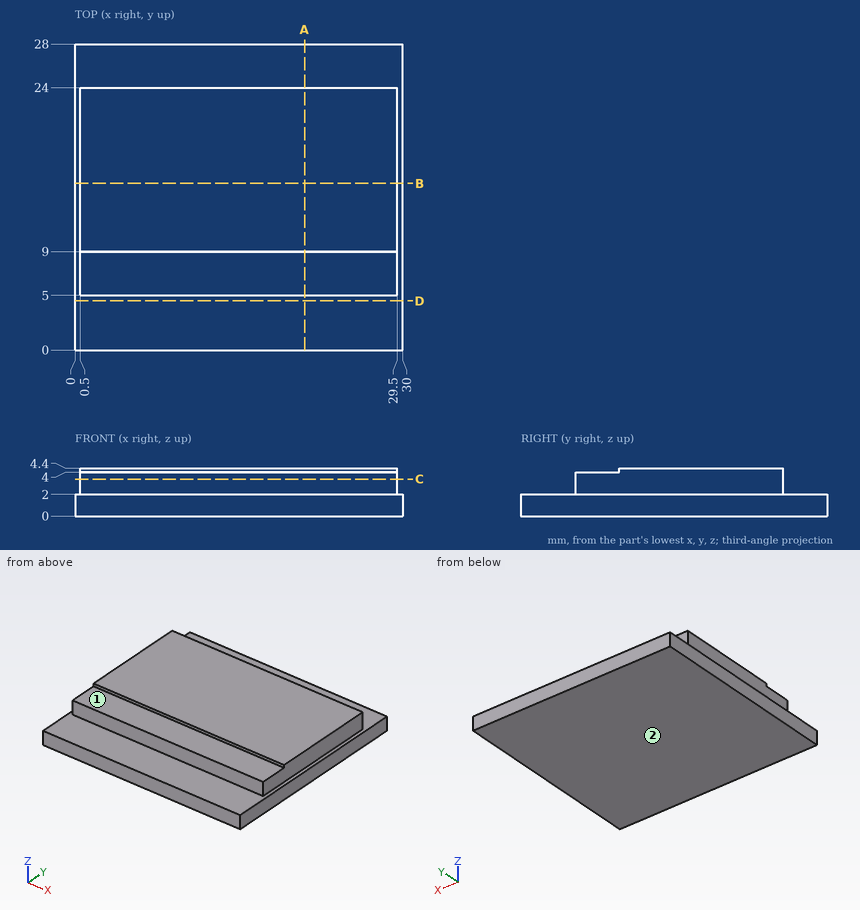
Print and shaded views of the part. All mm, measured from the part's lowest x, y and z. A direction names the side the tool comes from. Give positions to 0.01 mm unless a question says otherwise; leave off trailing zeros. Order: outer loops, then holes, each group sorted by start corner. A loop starts at its lowest first (then second) coordinate and runs counter-clockwise, first axis right, second up. Notation, with made-up numbers: (57, 69.25) - (116, 69.25) arc R6 ccw to (116, 77.25) - close; hole circle Ø2 at (27.5, -1). An arc over 180 degrees is marked (long way). Use a Markdown table: item, result.
1) Saw through at B-B on y = 15.25. List the corners of the cut face in (x, z), plus the area to 3 significant figures.
Checked values:
| item | result |
|---|---|
| outline | (0, 0) - (30, 0) - (30, 2) - (29.5, 2) - (29.5, 4.4) - (0.5, 4.4) - (0.5, 2) - (0, 2) - close |
| area | 130 mm² |
2) Probe L1, parallel to Z at x = 1.5, y = 4.75; L2, parallel to Y at x = 24, z = 3.05; L3, parallel to Y at x = 8.75, z = 4.1. List the from-to ranges inside material, lowest first. Write a range as from..to.
Checked values:
| item | result |
|---|---|
| L1 | 0..2 |
| L2 | 5..24 |
| L3 | 9..24 |
3) Saw through at C-C on z = 3.4. List the corners of the cut face in (x, y).
Checked values:
| item | result |
|---|---|
| outline | (0.5, 5) - (29.5, 5) - (29.5, 24) - (0.5, 24) - close |
4) 3-axis set-ups, long thin cutter, end or side, ignore diameter. For the marked faces 1 and 2: which of +Z, -Z, +X, -X, +Y, -Y reach the whole face in a straight line?
Checked values:
| item | result |
|---|---|
| face 1 | +Z, +X, -X, -Y |
| face 2 | -Z, +X, -X, +Y, -Y |
5) Saw through at A-A on x = 21. List the corners of the cut face in (y, z).
Checked values:
| item | result |
|---|---|
| outline | (0, 0) - (28, 0) - (28, 2) - (24, 2) - (24, 4.4) - (9, 4.4) - (9, 4) - (5, 4) - (5, 2) - (0, 2) - close |
6) Flat gauge pins, fed straight in: P1, Ø3, axis at x = 4.5, y = 21.5, coming from the -Z side; P2, Ø1, axis at y = 15, z = 4, coming from the +X side; P3, Ø0.7, axis at x = 10, z = 3.5, coming from the +Y side; P4, Ø1.9, axis at y = 12, z = 3, coming from the -X side. Where does each tip first touch, or does it go through?
Checked values:
| item | result |
|---|---|
| P1 | z = 0 |
| P2 | x = 29.5 |
| P3 | y = 24 |
| P4 | x = 0.5 |
7) Saw through at D-D on y = 4.5. List the corners of the cut face in (x, z).
Checked values:
| item | result |
|---|---|
| outline | (0, 0) - (30, 0) - (30, 2) - (0, 2) - close |
